from build123d import *

# Parameters (mm, degrees)
BOSS_EXTRUDE1_DEPTH = 100
SKETCH2_W           = 50
SKETCH2_H           = 50
BOSS_EXTRUDE2_DEPTH = 5
SKETCH3_R           = 3.5
CUT_EXTRUDE1_DEPTH  = 119.427192823
SKETCH4_R           = 5
CUT_EXTRUDE2_DEPTH  = 1


with BuildPart() as part:
    # Sketch1 → Boss-Extrude1 (new body)
    with BuildSketch(Plane(origin=(0, 0, 0), x_dir=(1, 0, 0), z_dir=(0, 1, 0))):
        Polygon((0, 0), (0, 20), (30, 0), align=None)
    extrude(amount=BOSS_EXTRUDE1_DEPTH)

    # Sketch2 → Boss-Extrude2 (add)
    with BuildSketch(Plane.XZ):
        with Locations((25, -25)):
            Rectangle(SKETCH2_W, SKETCH2_H)
    extrude(amount=-BOSS_EXTRUDE2_DEPTH)

    # Sketch3 → Cut-Extrude1 (cut, through all)
    with BuildSketch(Plane(origin=(0, 5, 0), x_dir=(1, 0, 0), z_dir=(0, 1, 0))):
        with Locations(Location((35, 35, 0), (0, 0, 270))):
            Circle(SKETCH3_R)
    extrude(amount=-CUT_EXTRUDE1_DEPTH, mode=Mode.SUBTRACT)

    # Sketch4 → Cut-Extrude2 (cut)
    with BuildSketch(Plane(origin=(0, 5, 0), x_dir=(1, 0, 0), z_dir=(0, 1, 0))):
        with Locations(Location((35, 35, 0), (0, 0, 270))):
            Circle(SKETCH4_R)
    extrude(amount=-CUT_EXTRUDE2_DEPTH, mode=Mode.SUBTRACT)


solid = part.part
Source: CAD feature listing. Evaluate the final solid. Frame: model axes, mm. A direction names the side the tool comes from. Give positions to 0.01 mm unless a question says otherwise; leave off trailing zeros. Write each loop counter-clockwise with the first axis right and the second up, starting at its lowest first coordinate (ties: lowest second). Pieces come first, ordered by that corner, then holes. Notation, with made-up numbers: (82, 7.5) -> (104, 7.5) arc R12 cw to (104, 26.5) -> close; hole circle Ø3 at (1, -18.75). An arc over 180 degrees is marked (long way). Return JSON: item names as keys, results as strings. Group by question number.
1. Access query for faces 4 (the face through (25, 2, -50)), 5 (the face through (32.8, 4, -31.7)). Directions: +Z, -Z, +X, -X, +Y, -Y. A direction counts if a zero-diameter tool reaches every point of the face in a straight line with its end or side. Return the directions, or none.
2. Section D-D, the plane y = 50. Output: boundary loops of the cut face in (x, z), then the cut area to 3 significant figures.
3. Mould query, pull axis Z, two halves, no side actions, for faces 1 (the face through (25, 5, -25)), 2 (the face through (35.22, 4.507, -39.995)), 3 (the face through (15, 52, -10)). Classes: +Z half, -Z half, draft (parallel to the pull), parting line (faces both ways), or undercut.
4. Material intervals for line 1 (X direction, y = 1.1, z = -35); line 2 (X direction, y = 4.6, z = -35); line 3 (Y direction, x = 33, z = -8), sorted ascending. Write a range as from..to.
5. Section B-B, the plane z = -35. Output: boundary loops of the cut face in (x, y).
6. Section C-C, the plane x = 27. Output: boundary loops of the cut face in (y, z).
7. Section A-A, the plane x = 35. Output: boundary loops of the cut face in (y, z), then the cut area to 3 significant figures.
8. Pin query (flat end, axial travel): pin 1 Ø4 at (x, y) = (25, 68) entering from +Z; pin 2 Ø8 at (x, z) = (22.5, -35) entering from +Y; pin 3 Ø8 at (x, z) = (35, -35) entering from +Y. Return the tip coordinate at first contact, or that it passes through.
Determined:
{
 "1": {"face 4": "-Z, +X, -X, +Y, -Y", "face 5": "+Y"},
 "2": {"outline": "(0, -20) -> (30, 0) -> (0, 0) -> close", "area": "300 mm2"},
 "3": {"face 1": "draft", "face 2": "undercut", "face 3": "-Z half"},
 "4": {"line 1": "x = 0..31.5, 38.5..50", "line 2": "x = 0..30, 40..50", "line 3": "y = 0..5"},
 "5": {"outline": "(0, 0) -> (31.5, 0) -> (31.5, 4) -> (30, 4) -> (30, 5) -> (0, 5) -> close; (38.5, 0) -> (50, 0) -> (50, 5) -> (40, 5) -> (40, 4) -> (38.5, 4) -> close"},
 "6": {"outline": "(0, -50) -> (5, -50) -> (5, -2) -> (100, -2) -> (100, 0) -> (0, 0) -> close"},
 "7": {"outline": "(0, -50) -> (5, -50) -> (5, -40) -> (4, -40) -> (4, -38.5) -> (0, -38.5) -> close; (0, -31.5) -> (4, -31.5) -> (4, -30) -> (5, -30) -> (5, 0) -> (0, 0) -> close", "area": "212 mm2"},
 "8": {"pin 1": "stops at z = 0", "pin 2": "stops at y = 5", "pin 3": "stops at y = 4"}
}
